Build history of the part. All positions in model axes, mm. Face numbers are marked on the shaded views. A direction names the side the tool comes from. Round coordinates to 2 decimals unless told otherwise and drop trailing zeros. Write each loop counter-clockwise with the first axis right and the second up, starting at its lowest first coordinate (ties: lowest second). Pieces come first, ordered by that corner, then holes.
1) Flat gauge pins, fed straight in: pin 1 (1.8 mm diameter, centred on x = 16, z = 15.5, fed in from +Y); pin 2 (7 mm diameter, centred on y = -4.5, z = 5, fed in from +X); pin 3 (10 mm diameter, centred on y = 5, z = 8.5, fed in from -X). Where does each tip first touch, or does it go through?
2) Which spindle directions (+Z, -Z, +X, -X, +Y, -Y) get a long thin tool onto all of the face, cutting with end or side? Do the marked faces 1, 2, 3, 4 and 5. Say none if no direction does.
3) Wall check: probe 1 along X at (y, z) = (11, -3.5); probe 2 along X at (y, z) = (6, 19); probe 3 along Y at (x, z) = (-14, -15.5). Give the ranges that are in metal, low to high.
4) Saw through at C-C (z = 15). Write the cut outline in (x, y).
5) Pull direction X, two halves, no side cores. Call the marked faces 6, 7 and 8: +X half, -X half, draft (parallel to the pull), parting line (faces both ways), or undercut.
6) Saw through at A-A (y = 17). Write the cut outline in (x, z), plus the area to 3 significant figures.
7) Saw through at B-B (x = -7). Write the cut outline in (y, z), plus the area to 3 significant figures.
8) Saw through at D-D (x = -16). Write the cut outline in (y, z), plus the area to 4 significant figures.
from build123d import *

# Parameters (mm, degrees)
PAD_DEPTH    = 22.5
SKETCH001_R  = 3
POCKET_DEPTH = 20


with BuildPart() as part:
    # Sketch → Pad (new body, symmetric)
    with BuildSketch(Plane.XY):
        with BuildLine():
            ThreePointArc((4.5, -6.614378), (0, 8), (-4.5, -6.614378))
            Line((-10, -13), (-4.5, -6.614378))
            Line((-10, -13), (-21, -13))
            Line((-21, -13), (-21, 11))
            Line((-21, 11), (-22.5, 12.5))
            Line((-22.5, 12.5), (-22.5, 18.5))
            Line((-22.5, 18.5), (-21, 20))
            Line((-21, 20), (-11.5, 20))
            Line((-11.5, 20), (-10, 18.5))
            Line((-10, 18.5), (10, 18.5))
            Line((10, 18.5), (11.5, 20))
            Line((11.5, 20), (21, 20))
            Line((21, 20), (22.5, 18.5))
            Line((22.5, 18.5), (22.5, 12.5))
            Line((22.5, 12.5), (21, 11))
            Line((21, 11), (21, -13))
            Line((21, -13), (10, -13))
            Line((10, -13), (4.5, -6.614378))
        make_face()
    extrude(amount=PAD_DEPTH, both=True)

    # Sketch001 → Pocket (cut)
    with BuildSketch(Plane.XZ.offset(-20)):
        with Locations((-16, 15)):
            Circle(SKETCH001_R)
        with Locations((16, 15)):
            Circle(SKETCH001_R)
        with Locations((16, -15)):
            Circle(SKETCH001_R)
        with Locations((-16, -15)):
            Circle(SKETCH001_R)
    extrude(amount=POCKET_DEPTH, mode=Mode.SUBTRACT)


solid = part.part
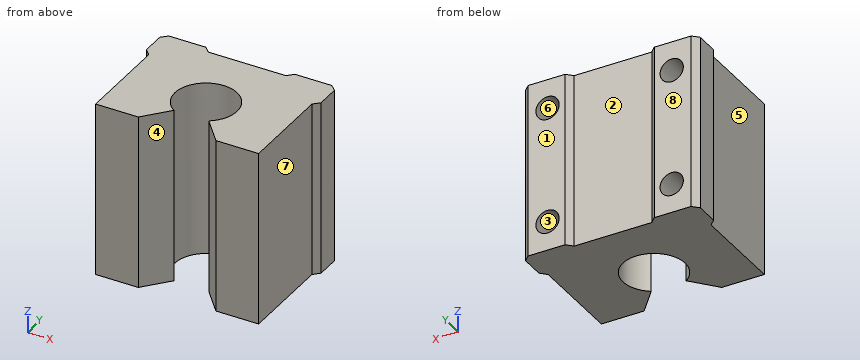
Evaluation:
1. pin 1: stops at y = 0
1. pin 2: stops at x = 21
1. pin 3: stops at x = -21
2. face 1: +Z, -Z, +X, -X, +Y
2. face 2: +Z, -Z, +Y
2. face 3: +Y
2. face 4: +Z, -Z, -Y
2. face 5: +Z, -Z, -X, -Y
3. probe 1: x = -21 to 21
3. probe 2: x = -21 to -5.29, 5.29 to 21
3. probe 3: y = -13 to 0
4. outline: (-22.5, 12.5) - (-21, 11) - (-21, -13) - (-10, -13) - (-4.5, -6.61) arc R8 cw (long way) to (4.5, -6.61) - (10, -13) - (21, -13) - (21, 11) - (22.5, 12.5) - (22.5, 18.5) - (21, 20) - (19, 20) - (19, 0) - (13, 0) - (13, 20) - (11.5, 20) - (10, 18.5) - (-10, 18.5) - (-11.5, 20) - (-13, 20) - (-13, 0) - (-19, 0) - (-19, 20) - (-21, 20) - (-22.5, 18.5) - close
5. face 6: undercut
5. face 7: +X half
5. face 8: draft
6. outline: (-22.5, -22.5) - (22.5, -22.5) - (22.5, 22.5) - (-22.5, 22.5) - close; hole circle Ø6 at (-16, -15); hole circle Ø6 at (-16, 15); hole circle Ø6 at (16, -15); hole circle Ø6 at (16, 15)
6. area: 1,910 mm2
7. outline: (-9.52, -22.5) - (-3.87, -22.5) - (-3.87, 22.5) - (-9.52, 22.5) - close; (3.87, -22.5) - (18.5, -22.5) - (18.5, 22.5) - (3.87, 22.5) - close
7. area: 912 mm2
8. outline: (-13, -22.5) - (20, -22.5) - (20, -18) - (0, -18) - (0, -12) - (20, -12) - (20, 12) - (0, 12) - (0, 18) - (20, 18) - (20, 22.5) - (-13, 22.5) - close
8. area: 1,245 mm2
